```python
from build123d import *

# Parameters (mm, degrees)
EXTRUDE_1_DEPTH           = 150
EXTRUDE_1_DEPTH_BACK      = 150
SKETCH_4_R                = 2.5
CUT_EXTRUDE_4_DEPTH       = 3
SKETCH_5_W                = 52
SKETCH_5_H                = 100
CUT_EXTRUDE_5_DEPTH       = 3
SKETCH_7_R                = 1.6
SKETCH_7_R_2              = 6.5
CUT_EXTRUDE_9_DEPTH       = 185.063533313
SKETCH_6_W                = 40
SKETCH_6_H                = 200
CUT_EXTRUDE_10_DEPTH      = 10
CUT_EXTRUDE_12_DEPTH      = 4
SKETCH_12_W               = 34
SKETCH_12_H               = 110
CUT_EXTRUDE_13_DEPTH      = 4
SKETCH_14_W               = 4.2
SKETCH_14_H               = 14
CUT_EXTRUDE_14_DEPTH      = 10
SKETCH_15_R               = 2
CUT_EXTRUDE_15_DEPTH      = 26
SKETCH_17_R               = 1.5
CUT_EXTRUDE_19_DEPTH      = 10
CUT_EXTRUDE_20_DEPTH      = 10
CUT_EXTRUDE_21_DEPTH      = 31
SKETCH_22_R               = 1.5
CUT_EXTRUDE_22_DEPTH      = 31
SKETCH_23_W               = 12
SKETCH_23_H               = 87.5
EXTRUDE_3_DEPTH           = 3
CUT_EXTRUDE_23_DEPTH      = 18
CUT_EXTRUDE_24_DEPTH      = 13
CUT_EXTRUDE_24_DEPTH_BACK = 4
SKETCH_25_R               = 1.5
SKETCH_26_R               = 2
CUT_EXTRUDE_25_DEPTH      = 10
CUT_EXTRUDE_29_DEPTH      = 10
CUT_EXTRUDE_30_DEPTH      = 3
SKETCH_34_W               = 3
SKETCH_34_H               = 40
CUT_EXTRUDE_31_DEPTH      = 10


with BuildPart() as part:
    # 草图1 → 凸台-拉伸1 (new, two sides: drawn at the far end of the back side and taken through both)
    with BuildSketch(Plane.XY.offset(-EXTRUDE_1_DEPTH_BACK)):
        Polygon((0, 4.173281966), (0, -73.826718034), (3, -73.826718034), (3, 1.173281966), (3, 3.173281966), (5, 3.173281966), (80, 3.173281966), (80, 6.173281966), (2, 6.173281966), (0, 6.173281966), align=None)
    extrude(amount=EXTRUDE_1_DEPTH + EXTRUDE_1_DEPTH_BACK)

    # 草图4 → 切除-拉伸4 (cut)
    with BuildSketch(Plane(origin=(0, 6.173281966, 0), x_dir=(1, 0, 0), z_dir=(0, 1, 0))):
        with Locations(Location((11.5, -72.5, 0), (0, 0, 180))):
            Circle(SKETCH_4_R)
        with Locations(Location((11.5, -127.5, 0), (0, 0, 180))):
            Circle(SKETCH_4_R)
    extrude(amount=-CUT_EXTRUDE_4_DEPTH, mode=Mode.SUBTRACT)

    # 草图5 → 切除-拉伸5 (cut)
    with BuildSketch(Plane(origin=(0, 6.173281966, 0), x_dir=(1, 0, 0), z_dir=(0, 1, 0))):
        with Locations((54, -100)):
            Rectangle(SKETCH_5_W, SKETCH_5_H)
    extrude(amount=-CUT_EXTRUDE_5_DEPTH, mode=Mode.SUBTRACT)

    # 草图7 → 切除-拉伸9 (cut, through all)
    with BuildSketch(Plane(origin=(3, 0, 0), x_dir=(0, 0, -1), z_dir=(1, 0, 0))):
        with Locations(Location((-54.5, -43.826718034, 0), (0, 0, 90))):
            Circle(SKETCH_7_R)
        with Locations(Location((-62.25, -30.403324275, 0), (0, 0, 90))):
            Circle(SKETCH_7_R)
        with Locations(Location((-62.25, -57.250111793, 0), (0, 0, 90))):
            Circle(SKETCH_7_R)
        with Locations(Location((-77.75, -30.403324275, 0), (0, 0, 90))):
            Circle(SKETCH_7_R)
        with Locations(Location((-77.75, -57.250111793, 0), (0, 0, 90))):
            Circle(SKETCH_7_R)
        with Locations(Location((-85.5, -43.826718034, 0), (0, 0, 90))):
            Circle(SKETCH_7_R)
        with Locations(Location((115.5, -43.826718034, 0), (0, 0, 90))):
            Circle(SKETCH_7_R)
        with Locations(Location((107.75, -30.403324275, 0), (0, 0, 90))):
            Circle(SKETCH_7_R)
        with Locations(Location((107.75, -57.250111793, 0), (0, 0, 90))):
            Circle(SKETCH_7_R)
        with Locations(Location((92.25, -30.403324275, 0), (0, 0, 90))):
            Circle(SKETCH_7_R)
        with Locations(Location((92.25, -57.250111793, 0), (0, 0, 90))):
            Circle(SKETCH_7_R)
        with Locations(Location((84.5, -43.826718034, 0), (0, 0, 90))):
            Circle(SKETCH_7_R)
        with Locations(Location((-70, -50.826718034, 0), (0, 0, 90))):
            Circle(SKETCH_7_R_2)
        with Locations(Location((100, -50.826718034, 0), (0, 0, 90))):
            Circle(SKETCH_7_R_2)
    extrude(amount=-CUT_EXTRUDE_9_DEPTH, mode=Mode.SUBTRACT)

    # 草图6 → 切除-拉伸10 (cut)
    with BuildSketch(Plane(origin=(0, 6.173281966, 0), x_dir=(1, 0, 0), z_dir=(0, 1, 0))):
        with Locations((60, 50)):
            Rectangle(SKETCH_6_W, SKETCH_6_H)
    extrude(amount=-CUT_EXTRUDE_10_DEPTH, mode=Mode.SUBTRACT)

    # 草图11 → 切除-拉伸12 (cut)
    with BuildSketch(Plane.ZY):
        Polygon((-128.345117246, -73.826718034), (-150, -73.826718034), (-150, 3.173281966), align=None)
    extrude(amount=-CUT_EXTRUDE_12_DEPTH, mode=Mode.SUBTRACT)

    # 草图12 → 切除-拉伸13 (cut)
    with BuildSketch(Plane(origin=(0, 6.173281966, 0), x_dir=(1, 0, 0), z_dir=(0, 1, 0))):
        with Locations((23, 95)):
            Rectangle(SKETCH_12_W, SKETCH_12_H)
    extrude(amount=-CUT_EXTRUDE_13_DEPTH, mode=Mode.SUBTRACT)

    # 草图14 → 切除-拉伸14 (cut)
    with BuildSketch(Plane.XZ.offset(-3.173281966)):
        with Locations((5.1, -103)):
            Rectangle(SKETCH_14_W, SKETCH_14_H)
    extrude(amount=-CUT_EXTRUDE_14_DEPTH, mode=Mode.SUBTRACT)

    # 草图15 → 切除-拉伸15 (cut)
    with BuildSketch(Plane(origin=(0, 6.173281966, 0), x_dir=(1, 0, 0), z_dir=(0, 1, 0))):
        with Locations(Location((32, -4.5, 0), (0, 0, 270))):
            Circle(SKETCH_15_R)
    extrude(amount=-CUT_EXTRUDE_15_DEPTH, mode=Mode.SUBTRACT)

    # 草图17 → 切除-拉伸19 (cut)
    with BuildSketch(Plane.XZ.offset(-3.173281966)):
        with Locations((23.690733746, 113.5)):
            Circle(SKETCH_17_R)
    extrude(amount=-CUT_EXTRUDE_19_DEPTH, mode=Mode.SUBTRACT)

    # 草图18 → 切除-拉伸20 (cut)
    with BuildSketch(Plane.ZY):
        Polygon((150, -73.826718034), (118.550084008, -73.826718034), (150, 0), align=None)
    extrude(amount=-CUT_EXTRUDE_20_DEPTH, mode=Mode.SUBTRACT)

    # 草图21 → 切除-拉伸21 (cut)
    with BuildSketch(Plane.ZY):
        Polygon((118.550084008, -73.826718034), (150, 0), (150, 6.173281966), (137.5, 6.173281966), (132.072189672, -6.568164552), (98.550084008, -73.826718034), align=None)
    extrude(amount=-CUT_EXTRUDE_21_DEPTH, mode=Mode.SUBTRACT)

    # 草图22 → 切除-拉伸22 (cut)
    with BuildSketch(Plane.ZY):
        with Locations(Location((-106, 3.173281966, 0), (0, 0, 270))):
            Circle(SKETCH_22_R)
        with Locations(Location((-100, 3.173281966, 0), (0, 0, 270))):
            Circle(SKETCH_22_R)
        with Locations(Location((-106, -1.826718034, 0), (0, 0, 270))):
            Circle(SKETCH_22_R)
        with Locations(Location((-100, -1.826718034, 0), (0, 0, 270))):
            Circle(SKETCH_22_R)
    extrude(amount=-CUT_EXTRUDE_22_DEPTH, mode=Mode.SUBTRACT)

    # 草图23 → 凸台-拉伸3 (add)
    with BuildSketch(Plane(origin=(0, 6.173281966, 0), x_dir=(1, 0, 0), z_dir=(0, 1, 0))):
        with Locations((34, -93.75)):
            Rectangle(SKETCH_23_W, SKETCH_23_H)
    extrude(amount=-EXTRUDE_3_DEPTH)

    # 草图24 → 切除-拉伸23 (cut)
    with BuildSketch(Plane.ZY.offset(-28)):
        Polygon((137.5, 6.173281966), (137.5, 3.173281966), (136.222010805, 3.173281966), align=None)
    extrude(amount=-CUT_EXTRUDE_23_DEPTH, mode=Mode.SUBTRACT)

    # 草图25 → 切除-拉伸24 (cut, two sides: drawn at the far end of the back side and taken through both)
    with BuildSketch(Plane(origin=(0, 6.173281966, 0), x_dir=(1, 0, 0), z_dir=(0, 1, 0)).offset(-CUT_EXTRUDE_24_DEPTH_BACK)):
        with Locations((32, -61)):
            Circle(SKETCH_25_R)
    extrude(amount=CUT_EXTRUDE_24_DEPTH + CUT_EXTRUDE_24_DEPTH_BACK, mode=Mode.SUBTRACT)

    # 草图26 → 切除-拉伸25 (cut)
    with BuildSketch(Plane.XZ.offset(-3.173281966)):
        with Locations((32, -25.5)):
            Circle(SKETCH_26_R)
    extrude(amount=-CUT_EXTRUDE_25_DEPTH, mode=Mode.SUBTRACT)

    # 草图31 → 切除-拉伸29 (cut)
    with BuildSketch(Plane(origin=(3, 0, 0), x_dir=(0, 0, -1), z_dir=(1, 0, 0))):
        Polygon((-38.550084008, -73.826718034), (-10.102483381, -23.826718034), (39.897516619, -23.826718034), (68.345117246, -73.826718034), align=None)
    extrude(amount=-CUT_EXTRUDE_29_DEPTH, mode=Mode.SUBTRACT)

    # 草图33 → 切除-拉伸30 (cut)
    with BuildSketch(Plane.ZY):
        Polygon((-150, 6.173281966), (-150, -87.897987577), (142.92942198, -91.593646071), (144.162869872, 6.173281966), align=None)
    extrude(amount=-CUT_EXTRUDE_30_DEPTH, mode=Mode.SUBTRACT)


with BuildPart() as cut_extrude_30_piece_1:
    # of the separate pieces the step leaves, piece 1, a body of its own (cut_extrude_30_pieces)
    add(part.part.solids().sort_by_distance((3, 3.173281966, 136.222010805))[0])


with BuildPart() as cut_extrude_30_piece_2:
    # of the separate pieces the step leaves, piece 2, a body of its own (cut_extrude_30_pieces)
    add(part.part.solids().sort_by_distance((6, 6.173281966, -110))[0])

    # 草图34 → 切除-拉伸31 (cut)
    with BuildSketch(Plane(origin=(0, 6.173281966, 0), x_dir=(1, 0, 0), z_dir=(0, 1, 0))):
        with Locations((4.5, 130)):
            Rectangle(SKETCH_34_W, SKETCH_34_H)
    extrude(amount=-CUT_EXTRUDE_31_DEPTH, mode=Mode.SUBTRACT)


solid = cut_extrude_30_piece_1.part
```
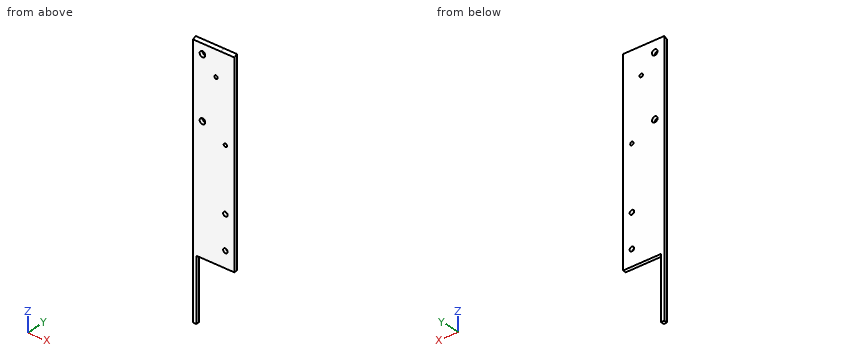
Could you check a few things on this model? Use its own coordinates, in mm. Give positions to 0.01 mm unless a question says otherwise; leave off trailing zeros. Write each loop counter-clockwise with the first axis right and the second up, starting at its lowest first coordinate (ties: lowest second). Pieces come first, ordered by that corner, then holes. Notation, with made-up numbers: (10, 37) - (42, 37) arc R30 cw to (42, 75) - close; hole circle Ø11 at (-34.5, -32.75). An arc over 180 degrees is marked (long way). One line per item, written item: value. Start each with the question number.
Item 1: I'm going to push flat-ended pins straight in: pin 1 (5 mm diameter, centred on x = 32, z = 4.5, fed in from -Y); pin 2 (1.5 mm diameter, centred on x = 16.5, y = 4.5, fed in from -Z); pin 3 (1.5 mm diameter, centred on y = 4, z = -71.5, fed in from +X). Where does each tip first touch, or does it pass through?
Item 2: Please list where these lines run through material, in increasing order: line 1 (Z direction, x = 11.5, y = 4.1); line 2 (Z direction, x = 11.5, y = 4.7); line 3 (X direction, y = 5.25, z = -54). Write a range as from..to.
Item 3: Imagine slicing it at C-C, the plane z = 127.5. List the corners of the cut face in (x, y) for me.
Item 4: Imagine slicing it at A-A, the plane z = -25.5. List the corners of the cut face in (x, y) for me, and give its area (3 significant figures).
Item 5: Imagine slicing it at D-D, the plane y = 3.9. List the corners of the cut face in (x, z) for me, and give its area (3 significant figures).
Item 6: Imagine slicing it at B-B, the plane x = 12. List the corners of the cut face in (y, z) for me.
Geometry says:
1. pin 1: y = 3.17
1. pin 2: z = -40
1. pin 3: x = 6
2. line 1: -40..70, 75..125, 130..136.62
2. line 2: -40..70, 75..125, 130..136.87
2. line 3: 3..6
3. outline: (3, 3.17) - (9, 3.17) - (9, 6.17) - (3, 6.17) - close; (14, 3.17) - (40, 3.17) - (40, 6.17) - (14, 6.17) - close
4. outline: (3, 3.17) - (30, 3.17) - (30, 6.17) - (3, 6.17) - close; (34, 3.17) - (40, 3.17) - (40, 6.17) - (34, 6.17) - close
4. area: 99.0 mm^2
5. outline: (3, -96) - (6, -96) - (6, -40) - (40, -40) - (40, 136.53) - (3, 136.53) - close; hole circle Ø5 at (11.5, 72.5); hole circle Ø5 at (11.5, 127.5); hole circle Ø3 at (23.69, 113.5); hole circle Ø4 at (32, -25.5); hole circle Ø4 at (32, 4.5); hole circle Ø3 at (32, 61)
5. area: 6,620 mm^2
6. outline: (3.17, -40) - (6.17, -40) - (6.17, 70.05) - (3.17, 70.05) - close; (3.17, 74.95) - (6.17, 74.95) - (6.17, 125.05) - (3.17, 125.05) - close; (3.17, 129.95) - (6.17, 129.95) - (6.17, 137.5) - (3.17, 136.22) - close
